from build123d import *

# Parameters (mm, degrees)
EXTRUDE_1_DEPTH = 3
CHAMFER_1_SIZE  = 0.3


with BuildPart() as part:
    # 草图1 → 凸台-拉伸1 (new body)
    with BuildSketch(Plane(origin=(0, 0, 0), x_dir=(1, 0, 0), z_dir=(0, 1, 0))):
        with BuildLine():
            Line((-3.5, 1.5), (3.5, 1.5))
            ThreePointArc((3.5, 1.5), (5, 0), (3.5, -1.5))
            Line((3.5, -1.5), (-3.5, -1.5))
            ThreePointArc((-3.5, -1.5), (-5, 0), (-3.5, 1.5))
        make_face()
    extrude(amount=EXTRUDE_1_DEPTH)

    # 倒角1
    chamfer_1_edges = [part.edges().sort_by_distance(p)[0] for p in [
        (5, 3, 0),
        (0, 3, -1.5),
        (-5, 3, 0),
        (0, 0, -1.5),
        (5, 0, 0),
        (0, 0, 1.5),
        (-5, 0, 0),
        (0, 3, 1.5),
    ]]
    chamfer(chamfer_1_edges, length=CHAMFER_1_SIZE)


solid = part.part
Source: CAD feature listing. Evaluate the final solid. Frame: model axes, mm. Give positions to 0.01 mm unless a question says otherwise; leave off trailing zeros. Write each loop counter-clockwise with the first axis right and the second up, starting at its lowest first coordinate (ties: lowest second). Pieces come first, ordered by that corner, then holes. Notation, with made-up numbers: (24, -30.75) -> (82, -30.75) arc R13 ccw to (82, -17.75) -> close; hole circle Ø7 at (49, 25). An arc over 180 degrees is marked (long way). Write item = value, one per line.
Q1. Cut plane A-A on x = -2.5. Return loops of the section in (y, z).
Here are the results:
outline = (0, -1.2) -> (0.3, -1.5) -> (2.7, -1.5) -> (3, -1.2) -> (3, 1.2) -> (2.7, 1.5) -> (0.3, 1.5) -> (0, 1.2) -> close
Q2. Line query: line 1 (X direction, y = 1.3, z = -0.8); line 2 (X direction, y = 2.5, z = 0.4); line 3 (Y direction, x = -4, z = -1.3). Output: solid intervals per line, ascending. Write a range as from..to.
Here are the results:
line_1 = -4.77..4.77
line_2 = -4.95..4.95
line_3 = 0.19..2.81
Q3. Cut plane B-B on y = 0.85. Return loops of the section in (x, z), then the cut area to 3 significant figures.
Here are the results:
outline = (-3.5, -1.5) -> (3.5, -1.5) arc R1.5 ccw to (3.5, 1.5) -> (-3.5, 1.5) arc R1.5 ccw to start
area = 28.1 mm²
